Geometry check sheet. Reference: the model listing, model coordinates, mm. A direction names the side the tool comes from. Coordinates: 2 decimals unless noted, no trailing zeros. Order: outer loops, then holes, each group sorted by start corner. A loop starts at its lowest first (then second) coordinate and runs counter-clockwise, first axis right, second up. Notation, with made-up numbers: (-19, -15) - (29, -15) arc R32 ccw to (29, 11) - close; hole circle Ø5 at (-29, 31.25). An arc over 180 degrees is marked (long way). Put each result on its own line as item: value.
from build123d import *

# Parameters (mm, degrees)
SKETCH1_R           = 3.175
BOSS_EXTRUDE3_DEPTH = 22.9108
SKETCH2_R           = 3.175
BOSS_EXTRUDE4_DEPTH = 5.588
BOSS_EXTRUDE5_DEPTH = 22.9108


with BuildPart() as part:
    # Sketch1 → Boss-Extrude3 (new body)
    with BuildSketch(Plane.XY):
        Polygon((-277.356124969, 264.279078056), (-301.486124969, 263.900029357), (-301.486124969, 241.343772944), (-277.356124969, 241.722821643), align=None)
        with Locations(Location((-285, 257.808220008, 0), (0, 0, 90))):
            Circle(SKETCH1_R, mode=Mode.SUBTRACT)
    extrude(amount=BOSS_EXTRUDE3_DEPTH)

    # Sketch2 → Boss-Extrude4 (add)
    with BuildSketch(Plane(origin=(0, 240.233117527, 23.037314684), x_dir=(1, 0, 0), z_dir=(0, 0.9954334818448494, 0.0954577562183399))):
        Polygon((-310.068865703, 46.86584189), (-306.799735692, -21.636195955), (-285.234279333, -20.607025396), (-288.503409344, 47.895012449), align=None)
        with Locations(Location((-298.922900855, 39.769089631, 0), (0, 0, 270))):
            Circle(SKETCH2_R, mode=Mode.SUBTRACT)
        with Locations(Location((-296.38024418, -13.510273137, 0), (0, 0, 270))):
            Circle(SKETCH2_R, mode=Mode.SUBTRACT)
    extrude(amount=-BOSS_EXTRUDE4_DEPTH)

    # Sketch5 → Boss-Extrude5 (add)
    with BuildSketch(Plane.XY.offset(22.9108)):
        Polygon((-301.486124969, 241.343772944), (-301.486124969, 240.2806727), (-277.356124969, 240.2806727), (-277.356124969, 241.722821643), align=None)
    extrude(amount=-BOSS_EXTRUDE5_DEPTH)


solid = part.part
Q1. Section check A-A on x = -283. Record the boundary of the cut face in (y, z).
Answer block:
outline: (240.28, 0) - (255.34, 0) - (255.34, 22.91) - (240.28, 22.91) - close; (260.27, 0) - (264.19, 0) - (264.19, 22.91) - (260.27, 22.91) - close
Q2. Section check D-D on y = 249.5. Record the boundary of the cut face in (x, z), then the cut area to 3 significant figures.
Answer block:
outline: (-301.49, 0) - (-277.36, 0) - (-277.36, 22.91) - (-301.49, 22.91) - close
area: 553 mm^2
Q3. Depth check by flat-ended pin: pin 1 Ø8 at (x, z) = (-295, 27) entering from -Y; pin 2 Ø8 at (x, y) = (-287.5, 257.5) entering from +Z; pin 3 Ø1.5 at (x, z) = (-303.5, -14.5) entering from -Y; pin 4 Ø6 at (y, z) = (248, -13) entering from -X. Enter the tip coordinate at first touch or a pass-through.
Answer block:
pin 1: stops at y = 233.86
pin 2: stops at z = 22.91
pin 3: stops at y = 238.15
pin 4: passes through
Q4. Access from +Z, -Z, +X, -X, +Y, -Y to the whole of each face (thin tool, end or side, straight path). Record for faces 1 (the flat face through (-301.486, 252, 12)), 2 (the flat face through (-290, 252, 22.911)), 3 (the flat face through (-277.356, 252, 12)).
Answer block:
face 1: +Z, -X, +Y
face 2: +Z, +X, -X, +Y
face 3: +Z, -Z, +X, +Y, -Y
Q5. Thickness scan on L1, parallel to Z at x = -285, y = 241; L2, parallel to Y at x = -286, z = 20; L3, parallel to Y at x = -285, z = 6. Record the ranges inside material, lowest first. Write a range as [from, to].
Answer block:
L1: z = [0, 22.91]
L2: y = [240.28, 254.79], [260.82, 264.14]
L3: y = [240.28, 254.63], [260.98, 264.16]
Q6. Draft check along X on faces 4 (the flat face through (-297.83, 235.97, 8.95)), 5 (the cylindrical face through (-295.43, 235.91, 39.24)), 6 (the flat face through (-299.1, 242, -24.4)), 7 (the cylindrical face through (-295.775, 241.327, -17.225)). Enter one of: pulls with the +X half, pulls with the -X half, needs draft (parallel to the pull), parting line crosses it, or undercut.
Answer block:
face 4: needs draft
face 5: undercut
face 6: pulls with the -X half
face 7: undercut
Q7. Section check B-B on z = 19.5. Record the boundary of the cut face in (x, y) (3 decimals), then the cut area to 3 significant figures.
Answer block:
outline: (-308.002, 240.572) - (-307.976, 234.959) - (-286.362, 234.959) - (-286.386, 240.281) - (-277.356, 240.281) - (-277.356, 264.279) - (-301.486, 263.9) - (-301.486, 240.572) - close; hole circle Ø6.35 at (-285, 257.808)
area: 660 mm^2
Q8. Section check C-C on x = -295. Record the boundary of the cut face in (y, z).
Answer block:
outline: (232.66, 43.48) - (233.11, 38.8) - (238.67, 39.33) - (238.22, 44.01) - close; (233.65, 33.11) - (239.21, -24.86) - (244.78, -24.33) - (242.44, 0) - (264, 0) - (264, 22.91) - (240.28, 22.91) - (240.28, 22.54) - (239.22, 33.64) - close
